```python
from build123d import *

# Parameters (mm, degrees)
SKETCH2_R               = 19.762
SKETCH2_W               = 12.9032
SKETCH2_H               = 19.685
BOSS_EXTRUDE1_DEPTH     = 3.175
F_6_CLEARANCE_HOLE1_D   = 3.6576
FILLET1_R               = 0.635
F_1_4_CLEARANCE_HOLE1_D = 6.5278


with BuildPart() as part:
    # Sketch2 → Boss-Extrude1 (new body)
    with BuildSketch(Plane.XY):
        Polygon((105.5, 66.04), (-46.9, 66.04), (-46.9, -40.64), (-13.062, -40.64), (-13.062, -12.878), (18.762, -12.878), (18.762, -40.64), (46.9, -40.64), (105.5, 40.64), align=None)
        with Locations((0.58, 19.04)):
            Circle(SKETCH2_R, mode=Mode.SUBTRACT)
        with Locations((46.9, 19.04)):
            Rectangle(SKETCH2_W, SKETCH2_H, mode=Mode.SUBTRACT)
    extrude(amount=BOSS_EXTRUDE1_DEPTH)

    # #6 Clearance Hole1 (through all)
    with Locations(Plane.XY.offset(3.175)):
        with Locations((-15.42, 35.04), (16.58, 35.04), (16.58, 3.04), (-15.42, 3.04), (-18.198, -26.14)):
            Hole(F_6_CLEARANCE_HOLE1_D / 2)

    # Fillet1
    fillet1_edges = [part.edges().sort_by_distance(p)[0] for p in [
        (18.762, -40.64, 1.5875),
        (18.762, -12.878, 1.5875),
        (-13.062, -12.878, 1.5875),
        (-13.062, -40.64, 1.5875),
    ]]
    fillet(fillet1_edges, radius=FILLET1_R)

    # 1/4 Clearance Hole1 (through all)
    with Locations(Plane.XY.offset(3.175)):
        with Locations((-34.2, -22.86), (-8.8, 53.34), (92.8, 53.34), (-34.2, 27.94)):
            Hole(F_1_4_CLEARANCE_HOLE1_D / 2)


solid = part.part
```
Verification items for the finished model (mm, model axes). A direction names the side the tool comes from. Coordinates: 2 decimals unless noted, no trailing zeros. Order: outer loops, then holes, each group sorted by start corner. A loop starts at its lowest first (then second) coordinate and runs counter-clockwise, first axis right, second up. Notation, with made-up numbers: (-26, 62.5) -> (28, 62.5) arc R24 cw to (28, 99.5) -> close; hole circle Ø4 at (42, 18). An arc over 180 degrees is marked (long way). Put each result on its own line as item: value. Start each with the question number.
1) Cross-section at D-D (x = 0.58). Enter the section's corners in (y, z) (3 decimals), plus the area to 3 significant figures.
2) Material ranges on L1, parallel to X at y = 24, z = 0.5; L2, parallel to Y at x = -15.42, z = 2.1; L3, parallel to Y at x = -8.8, z = 2.2, recorded low to high.
3) Cross-section at A-A (x = -34.2). Enter the section's corners in (y, z) (3 decimals).
4) Tool access check on faces 4 (the flat face through (18.762, -27, 2)), 5 (the flat face through (33, -40.64, 2)), 6 (the flat face through (53.352, 19, 2)). Record the directions out of +Z, -Z, +X, -X, +Y, -Y that give a thin tool (end or side, any length) a straight path to the whole face; none if there is none.
5) Go/stop test with flat-tipped pins: pin 1 (1 mm diameter, centred on y = -25, z = 2, fed in from +X); pin 2 (1 mm diameter, centred on x = -3.5, z = 1.5, fed in from -Y). Record where each tip stops, or that it passes through.
6) Release check for a two-part mould opening along X. For faces 1 (the cylindrical face through (16.976, 33.255, 1.565)), 2 (the flat face through (-46.9, 13, 2)), 3 (the flat face through (105.5, 53, 2)) record: pulls with the +X half, pulls with the -X half, needs draft (parallel to the pull), parting line crosses it, or undercut.
7) Cross-section at B-B (z = 0.6). State how many separate pieces and enclosed holes the cut face has, plus the area to 3 significant figures.
8) Cross-section at C-C (y = 19.04). Enter the section's corners in (x, z) (3 decimals).
Geometry check:
1. outline: (-12.878, 0) -> (-0.722, 0) -> (-0.722, 3.175) -> (-12.878, 3.175) -> close; (38.802, 0) -> (66.04, 0) -> (66.04, 3.175) -> (38.802, 3.175) -> close
1. area: 125 mm^2
2. L1: x = -46.9 to -18.55, 19.71 to 40.45, 53.35 to 93.5
2. L2: y = -40.64 to 1.21, 4.87 to 7.44, 30.64 to 33.21, 36.87 to 66.04
2. L3: y = -12.88 to 1.65, 36.43 to 50.08, 56.6 to 66.04
3. outline: (-40.64, 0) -> (-26.124, 0) -> (-26.124, 3.175) -> (-40.64, 3.175) -> close; (-19.596, 0) -> (24.676, 0) -> (24.676, 3.175) -> (-19.596, 3.175) -> close; (31.204, 0) -> (66.04, 0) -> (66.04, 3.175) -> (31.204, 3.175) -> close
4. face 4: +Z, -Z, -Y
4. face 5: +Z, -Z, +X, -X, -Y
4. face 6: +Z, -Z
5. pin 1: stops at x = 58.54
5. pin 2: stops at y = -12.88
6. face 1: undercut
6. face 2: pulls with the -X half
6. face 3: pulls with the +X half
7. separate pieces: 1
7. enclosed holes: 11
7. area: 11,300 mm^2
8. outline: (-46.9, 0) -> (-19.182, 0) -> (-19.182, 3.175) -> (-46.9, 3.175) -> close; (20.342, 0) -> (40.448, 0) -> (40.448, 3.175) -> (20.342, 3.175) -> close; (53.352, 0) -> (89.927, 0) -> (89.927, 3.175) -> (53.352, 3.175) -> close
